```python
from build123d import *

# Parameters (mm, degrees)
BOSS_EXTRUDE1_DEPTH = 73.3796339
SKETCH2_R           = 7
BOSS_EXTRUDE2_DEPTH = 1
CUT_EXTRUDE1_START  = -10
CUT_EXTRUDE1_DEPTH  = 10


with BuildPart() as part:
    # Sketch1 → Boss-Extrude1 (new body)
    with BuildSketch(Plane.XY):
        with BuildLine():
            Line((3.5, -1.936491673), (3.5, 1.936491673))
            ThreePointArc((3.5, 1.936491673), (-4, 0), (3.5, -1.936491673))
        make_face()
    extrude(amount=-BOSS_EXTRUDE1_DEPTH)

    # Sketch2 → Boss-Extrude2 (add)
    with BuildSketch(Plane.XY):
        Circle(SKETCH2_R)
    extrude(amount=BOSS_EXTRUDE2_DEPTH)

    # Sketch3 → Cut-Extrude1 (cut)
    with BuildSketch(Plane(origin=(0, 0, -73.3796339), x_dir=(-1, 0, 0), z_dir=(0, 0, -1)).offset(CUT_EXTRUDE1_START)):
        with BuildLine():
            Line((-3.5, 1.936491673), (3.5, 1.936491673))
            ThreePointArc((3.5, 1.936491673), (0, 4), (-3.5, 1.936491673))
        make_face()
        with BuildLine():
            Line((-3.5, -1.936491673), (3.5, -1.936491673))
            ThreePointArc((3.5, -1.936491673), (0, -4), (-3.5, -1.936491673))
        make_face()
    extrude(amount=CUT_EXTRUDE1_DEPTH, mode=Mode.SUBTRACT)


solid = part.part
```
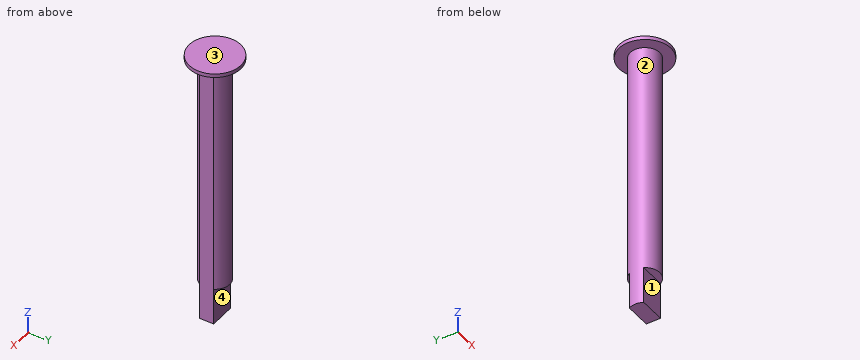
Check sheet for the modelled part. Datum: model origin and axes. Units: mm. Face numbers are marked on the shaded views. A direction names the side the tool comes from. Round coordinates to 2 decimals unless told otherwise and drop trailing zeros. Loops run counter-clockwise (first coordinate to the right, second up) from the corner with the lowest first, then second, coordinate; pieces in that order, holes last. Notation, with made-up numbers: (-8.75, 20.25) - (44.25, 20.25) arc R36 cw to (44.25, 55.25) - close; hole circle Ø7 at (76.5, -6). An arc over 180 degrees is marked (long way). Write item = value, one per line. Start each with the question number.
Q1. Access from +Z, -Z, +X, -X, +Y, -Y to the whole of each face (thin tool, end or side, straight path). Record for the marked faces 1 and 2.
Q2. Section check C-C (z = -68). Record the boundary of the cut face in (x, y).
Q3. Release check for a two-part mould opening along Z. For the marked faces 3 and 4 record: pulls with the +Z half, pulls with the -Z half, needs draft (parallel to the pull), parting line crosses it, or undercut.
Q4. Depth check by flat-ended pin: P1, Ø5, axis at x = -5.5, z = -19.5, coming from the -Y side; P2, Ø3, axis at y = 0, z = -31, coming from the +X side; P3, Ø6, axis at x = -5, z = -11, coming from the +Y side. Enter the tip coordinate at first touch or a pass-through.
Q5. Section check B-B (y = 0). Record the boundary of the cut face in (x, z).
Q6. Thickness scan on L1, parallel to Z at x = -1.5, y = 3.5; L2, parallel to Z at x = -5, y = -4.5; L3, parallel to Y at x = -2, z = -68.5. Record the ranges inside material, lowest first.
Q7. Section check A-A (x = 0). Record the boundary of the cut face in (y, z).
Q8. Section check D-D (y = -3). Record the boundary of the cut face in (x, z).
Derived:
q1.face_1 = -Z, +X, -X, -Y
q1.face_2 = -Z
q2.outline = (-3.5, -1.94) - (3.5, -1.94) - (3.5, 1.94) - (-3.5, 1.94) arc R4 ccw to start
q3.face_3 = pulls with the +Z half
q3.face_4 = needs draft
q4.P1 = -2.65
q4.P2 = 3.5
q4.P3 = 3.46
q5.outline = (-7, 0) - (-4, 0) - (-4, -73.38) - (3.5, -73.38) - (3.5, 0) - (7, 0) - (7, 1) - (-7, 1) - close
q6.L1 = -63.38 to 1
q6.L2 = 0 to 1
q6.L3 = -1.94 to 1.94
q7.outline = (-7, 0) - (-4, 0) - (-4, -63.38) - (-1.94, -63.38) - (-1.94, -73.38) - (1.94, -73.38) - (1.94, -63.38) - (4, -63.38) - (4, 0) - (7, 0) - (7, 1) - (-7, 1) - close
q8.outline = (-6.32, 0) - (-2.65, 0) - (-2.65, -63.38) - (2.65, -63.38) - (2.65, 0) - (6.32, 0) - (6.32, 1) - (-6.32, 1) - close
